Autodesk Inventor part; units mm, degrees
ref_plane "YZ Plane" through (0, 0, 0) normal (1, 0, 0) x (0, 1, 0)
ref_plane "XZ Plane" through (0, 0, 0) normal (0, 1, 0) x (-1, 0, 0)
ref_plane "XY Plane" through (0, 0, 0) normal (0, 0, 1) x (1, 0, 0)
sketch "Sketch1" plane through (0, 0, 0) normal (0, 0, 1) x (1, 0, 0)
  line L0 (0, 46.188) -> (40, 23.094)
  line L1 (40, 23.094) -> (40, -23.094)
  line L2 (40, -23.094) -> (0, -46.188)
  line L3 (0, -46.188) -> (-40, -23.094)
  line L4 (-40, -23.094) -> (-40, 23.094)
  line L5 (-40, 23.094) -> (0, 46.188)
  line L6 (0, 38.1051) -> (33, 19.0526)
  line L7 (33, 19.0526) -> (33, -19.0526)
  line L8 (33, -19.0526) -> (0, -38.1051)
  line L9 (0, -38.1051) -> (-33, -19.0526)
  line L10 (-33, -19.0526) -> (-33, 19.0526)
  line L11 (-33, 19.0526) -> (0, 38.1051)
  point P0 (0, 0)
  point P1 (0, 0)
  dimension "d1" = 66
  dimension "d36" = 7
extrude "Extrusion1" add sketch "Sketch1" along normal blind 100
sketch "Sketch7" plane through (0, 0, 100) normal (0, 0, 1) x (1, 0, 0)
  circle A0 centre (0, 0) radius 33
  line L0 (-33, 19.0526) -> (0, 38.1051)
  line L1 (33, 19.0526) -> (33, -19.0526)
  line L2 (33, -19.0526) -> (0, -38.1051)
  line L3 (0, -38.1051) -> (-33, -19.0526)
  line L4 (-33, -19.0526) -> (-33, 19.0526)
  line L5 (-33, 19.0526) -> (0, 38.1051)
  line L6 (0, 38.1051) -> (33, 19.0526)
  line L7 (40, 23.094) -> (0, 46.188)
  line L8 (0, 46.188) -> (-40, 23.094)
  line L9 (-40, 23.094) -> (-40, -23.094)
  line L10 (-40, -23.094) -> (0, -46.188)
  line L11 (0, -46.188) -> (40, -23.094)
  line L12 (40, -23.094) -> (40, 23.094)
extrude "Extrusion6" add sketch "Sketch7" against normal up to surface (100 mm away) from surface at 0 contours L1 L2 A0 | A0 L6 L1 | A0 L0 L6 | L2 L3 A0 | A0 L4 L0 | L3 L4 A0
sketch "Sketch2" plane through (40, -23.094, 0) normal (1, 0, 0) x (0, 0, -1)
  line L0 (-91, 16.0229) -> (-96, 30.1651) construction
  line L1 (-100, 0) -> (-100, 46.188)
  circle A0 centre (-96, 30.1651) radius 2.5
  circle A1 centre (-91, 16.0229) radius 2.5
  line L2 (-4, 16.0229) -> (-9, 30.1651) construction
  circle A2 centre (-9, 30.1651) radius 2.5
  circle A3 centre (-4, 16.0229) radius 2.5
  line L3 (0, 46.188) -> (0, 0)
  point P0 (0, 23.094)
  point P1 (-93.5, 23.094)
  point P2 (-100, 23.094)
  point P3 (-6.5, 23.094)
  point P4 (0, 23.094)
  dimension "d4" = 15
  dimension "d6" = 5
  dimension "d7" = 5
  dimension "d28" = 6.5
  dimension "d29" = 5
  dimension "d30" = 15
  dimension "d31" = 5
  dimension "d32" = 5
  dimension "d34" = 5
  dimension "d35" = 6.5
extrude "Extrusion2" cut sketch "Sketch2" against normal blind 30
pattern_circular "Circular Pattern1" count 6 over 360 about axis through (0, 0, -10) along (0, 0, 1) of "Extrusion2"
sketch "Sketch8" plane through (0, 0, 100) normal (0, 0, 1) x (1, 0, 0)
  line L0 (0, 38.1051) -> (33, 19.0526)
  line L1 (33, 19.0526) -> (33, -19.0526)
  line L2 (33, -19.0526) -> (0, -38.1051)
  line L3 (0, -38.1051) -> (-33, -19.0526)
  line L4 (-33, -19.0526) -> (-33, 19.0526)
  line L5 (-33, 19.0526) -> (0, 38.1051)
  point P0 (0, 0)
  point P1 (0, 0)
  point P2 (0, 46.188)
  dimension "d39" = 66
extrude "Extrusion7" cut sketch "Sketch8" against normal blind 15
sketch "Sketch9" plane through (0, 0, 0) normal (0, 0, -1) x (-1, 0, 0)
  arc A0 (16.5, 28.5788) -> (-16.5, 28.5788) centre (0, 0) ccw
  line L0 (0, 38.1051) -> (-16.5, 28.5788)
  line L1 (16.5, 28.5788) -> (0, 38.1051)
  arc A1 (33, 0) -> (16.5, 28.5788) centre (0, 0) ccw
  line L2 (33, 19.0526) -> (16.5, 28.5788)
  line L3 (33, 0) -> (33, 19.0526)
  arc A2 (16.5, -28.5788) -> (33, 0) centre (0, 0) ccw
  line L4 (33, -19.0526) -> (33, 0)
  line L5 (16.5, -28.5788) -> (33, -19.0526)
  arc A3 (-16.5, -28.5788) -> (16.5, -28.5788) centre (0, 0) ccw
  line L6 (0, -38.1051) -> (16.5, -28.5788)
  line L7 (-16.5, -28.5788) -> (0, -38.1051)
  arc A4 (-33, 0) -> (-16.5, -28.5788) centre (0, 0) ccw
  line L8 (-33, -19.0526) -> (-16.5, -28.5788)
  line L9 (-33, 0) -> (-33, -19.0526)
  arc A5 (-16.5, 28.5788) -> (-33, 0) centre (0, 0) ccw
  line L10 (-33, 19.0526) -> (-33, 0)
  line L11 (-16.5, 28.5788) -> (-33, 19.0526)
extrude "Extrusion8" cut sketch "Sketch9" against normal blind 15 contours A0 L0 L1 | L2 L3 A1 | A5 L10 L11 | L4 L5 A2 | A4 L8 L9 | L6 L7 A3
sketch "Sketch10" plane through (40, -23.094, 0) normal (0.5, -0.866, 0) x (0.866, 0.5, 0)
  circle A0 centre (-10, 50) radius 2
  line L0 (0, 0) -> (0, 100)
  point P0 (-23.094, 0)
  point P1 (0, 50)
  dimension "d44" = 4
  dimension "d45" = 10
extrude "Extrusion9" cut sketch "Sketch10" against normal blind 15
sketch "Sketch11" plane through (-40, -23.094, 0) normal (-1, 0, 0) x (0, 0, 1)
  circle A0 centre (50, 36.188) radius 2.5
  line L0 (0, 46.188) -> (100, 46.188)
  point P0 (0, 23.094)
  point P1 (50, 46.188)
  dimension "d48" = 5
  dimension "d49" = 10
extrude "Extrusion10" cut sketch "Sketch11" against normal blind 15
properties part number "A01" material "ABS Plastic"
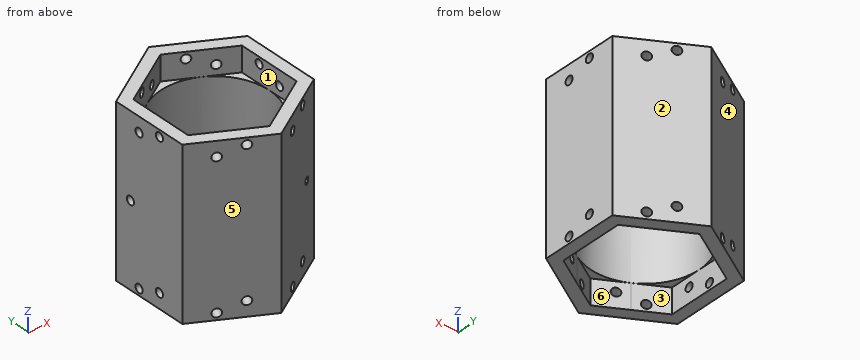
Design review of the part built by this model. Coordinates are the model's own, in mm. Face numbers are marked on the shaded views. A direction names the side the tool comes from. Coordinates: 2 decimals unless noted, no trailing zeros. Order: outer loops, then holes, each group sorted by start corner. A loop starts at its lowest first (then second) coordinate and runs counter-clockwise, first axis right, second up. Notation, with made-up numbers: M -24,31.5 L -3,31.5 A21 ccw -3,49.5 Z; hole C -10,-19.75 d8. An arc over 180 degrees is marked long. Answer as a JSON object with one key per item and string values. Group by question number.
1) Wall thickness on L1, parallel to Z at x = 35.5, y = 7; L2, parallel to X at y = -18.5, z = 94; L3, parallel to X at y = 17, z = 29: over which ranges is each line inside the solid? List them lowest first.
2) Tool access review of the marked faces 1, 2 and 3: name each direction out of +Z, -Z, +X, -X, +Y, -Y from which nothing blocks a thin tool from reaching the whole face with its end or side.
3) Add section C-C, the plane y = -3. Write out the cut boundary in (x, z).
4) Mouldability with a two-part tool opening along Y and no side actions: class the marked faces 4, 5 and 6 as pulls with the +Y half, pulls with the -Y half, needs draft (parallel to the pull), parting line crosses it, or undercut.
5) Add section A-A, the plane z = 17. Write out the cut boundary in (x, y), then the cut area to 3 significant figures.
6) Add section B-B, the plane x = 35.5. Write out the cut boundary in (y, z), then the cut area to 3 significant figures.
7) Add section D-D, the plane z = 50. Write out the cut boundary in (x, y), then the cut area to 3 significant figures.
8) For pin 1 (6 mm diameter, centred on x = 5.5, z = 37, fed in from -Y); pin 2 (10 mm diameter, centred on y = -34.5, z = 63.5, fed in from -X); pin 3 (12 mm diameter, centred on x = 25.5, z = 71.5, fed in from -Y); pin 4 (5 mm diameter, centred on x = -24, y = 18, fed in from -Z), all flat-tipped, find the tip position at first contact; note any pin that passes through.
Computed values:
{
 "1": {"L1": "z = 0 to 6.5, 11.5 to 93.5, 98.5 to 100", "L2": "x = -40 to -33, 33 to 40", "L3": "x = -40 to -28.28, 28.28 to 40"},
 "2": {"face 1": "+Z", "face 2": "+Z, -Z, +X, +Y", "face 3": "-Z"},
 "3": {"outline": "M -40,0 L -33,0 L -33,15 L -32.86,15 L -32.86,85 L -33,85 L -33,100 L -40,100 Z; M 32.86,15 L 33,15 L 33,0 L 40,0 L 40,100 L 33,100 L 33,85 L 32.86,85 Z"},
 "4": {"face 4": "pulls with the +Y half", "face 5": "pulls with the -Y half", "face 6": "undercut"},
 "5": {"outline": "M -40,-23.09 L 0,-46.19 L 40,-23.09 L 40,23.09 L 0,46.19 L -40,23.09 Z; hole C 0,0 d66", "area": "2,120 mm^2"},
 "6": {"outline": "M -25.69,0 L 25.69,0 L 25.69,100 L -25.69,100 Z; hole C -7.07,4 d5; hole C -7.07,91 d5; hole C 7.07,9 d5; hole C 7.07,96 d5", "area": "5,060 mm^2"},
 "7": {"outline": "M -40,-23.09 L 0,-46.19 L 29.61,-29.09 L 25.15,-21.37 A33 cw -31.25,10.59 L -40,10.59 Z; M -40,15.59 L -29.08,15.59 A33 cw long 27.74,-17.87 L 33.07,-27.09 L 40,-23.09 L 40,23.09 L 0,46.19 L -40,23.09 Z", "area": "2,030 mm^2"},
 "8": {"pin 1": "stops at y = -44.74", "pin 2": "stops at x = -28.9", "pin 3": "stops at y = -34.93", "pin 4": "passes through"}
}
